Autodesk Inventor part; units mm, degrees
ref_plane "YZ Plane" through (0, 0, 0) normal (1, 0, 0) x (0, 1, 0)
ref_plane "XZ Plane" through (0, 0, 0) normal (0, 1, 0) x (-1, 0, 0)
ref_plane "XY Plane" through (0, 0, 0) normal (0, 0, 1) x (1, 0, 0)
sketch "Sketch1" plane through (0, 0, 0) normal (0, 1, 0) x (-1, 0, 0)
  line L0 (3, 9) -> (-3, 9)
  line L1 (-3, 9) -> (-3, -9)
  line L2 (-3, -9) -> (3, -9)
  line L3 (3, -9) -> (3, 9)
  line L4 (3, 9) -> (-3, -9) construction
  line L5 (-3, 9) -> (3, -9) construction
  circle A0 centre (0, 9) radius 3
  circle A1 centre (0, -9) radius 3
  line L6 (-3, -9) -> (-7, -9)
  line L7 (-7, -9) -> (-7, -5)
  line L8 (-7, -5) -> (-7, -3)
  line L9 (-7, -3) -> (-3, -3)
  line L10 (-7, -3) -> (-7, -6)
  circle A2 centre (-7, -6) radius 3
  line L11 (-3, -3) -> (-3, -9)
  point P0 (0, 0)
  dimension "d0" = 6
  dimension "d1" = 18
  dimension "d2" = 6
  dimension "d4" = 6
  dimension "d5" = 4
  dimension "d6" = 4
  dimension "d7" = 2
  dimension "d10" = 3
  dimension "d11" = 6
extrude "Extrusion1" add sketch "Sketch1" along normal blind 1.5 contours A0 L0 | L0 A0 | L3 A1 L1 A0 | A1 L2 | L2 A1 | A2 L7 L8 | L8 L7 A2
sketch "Sketch2" plane through (0, 1.5, 0) normal (0, 1, 0) x (1, 0, 0)
  line L0 (3, -9) -> (3, 9)
  arc A0 (3, 9) -> (-3, 9) centre (0, 9) ccw
  line L1 (-3, 9) -> (-3, -9)
  arc A1 (-3, -9) -> (3, -9) centre (0, -9) ccw
  circle A2 centre (0, 9) radius 1.5
  circle A3 centre (0, -9) radius 1.5
  line L2 (3, 9) -> (7, 9)
  line L3 (7, 9) -> (7, 3)
  line L4 (7, 3) -> (3, 3)
  line L5 (3, 3) -> (3, 9)
  point P0 (0, 0)
  dimension "d14" = 3
  dimension "d15" = 3
  dimension "d16" = 4
  dimension "d17" = 6
extrude "Extrusion2" cut sketch "Sketch2" against normal blind 1.5 contours L0 L2 L3 L4 | A2 | A3
sketch "Sketch3" plane through (0, 1.5, 0) normal (0, 1, 0) x (1, 0, 0)
  line L0 (3, -9) -> (3, 9)
  arc A0 (3, 9) -> (-3, 9) centre (0, 9) ccw
  line L1 (-3, 9) -> (-3, -9)
  line L2 (3, 9) -> (7, 9)
  line L3 (7, 9) -> (7, 3)
  line L4 (7, 3) -> (3, 3)
  line L5 (3, 3) -> (3, 9)
  point P0 (0, 0)
  dimension "d20" = 4
  dimension "d21" = 6
  dimension "d22" = 4
extrude "Extrusion3" add sketch "Sketch3" against normal blind 1.5
sketch "Sketch4" plane through (0, 1.5, 0) normal (0, 1, 0) x (1, 0, 0)
  arc A0 (7, 3) -> (7, 9) centre (7, 6) ccw
  circle A1 centre (7, 6) radius 1.5
  point P0 (0, 0)
  dimension "d25" = 3
extrude "Extrusion4" cut sketch "Sketch4" against normal blind 1.5
sketch "Sketch5" plane through (0, 0, 0) normal (0, -1, 0) x (1, 0, 0)
  circle A0 centre (7, -6) radius 1.5
  circle A1 centre (0, 9) radius 1.5
  circle A2 centre (0, -9) radius 1.5
  arc A3 (7, -9) -> (7, -3) centre (7, -6) ccw
  arc A4 (3, 9) -> (-3, 9) centre (0, 9) ccw
  arc A5 (-3, -9) -> (3, -9) centre (0, -9) ccw
  circle A6 centre (0, 9) radius 0.1
  circle A7 centre (0, -9) radius 0.1
  circle A8 centre (7, -6) radius 0.1
  point P0 (0, 0)
  dimension "d28" = 0.2
  dimension "d29" = 0.2
  dimension "d30" = 0.2
extrude "Extrusion5" add sketch "Sketch5" against normal blind 1.5
properties part number "tahlo3_sablona"
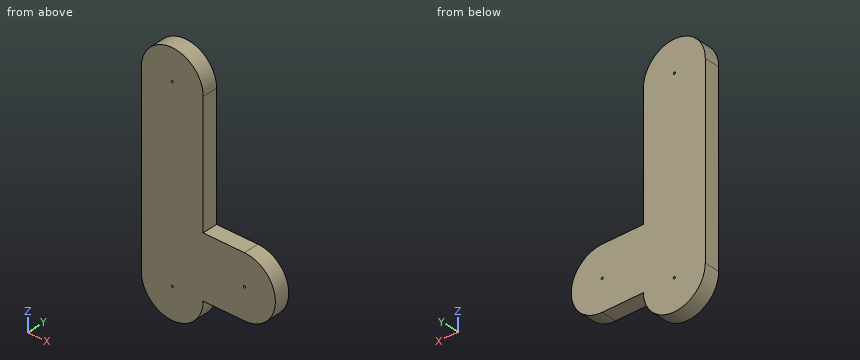
Read the model definition and answer for the solid it produces. Units are mm, in the model's axes. Coordinates: 2 decimals unless noted, no trailing zeros. Loops run counter-clockwise (first coordinate to the right, second up) from the corner with the lowest first, then second, coordinate; pieces in that order, holes last. Notation, with made-up numbers: (68.5, -0.75) - (87.5, -0.75) arc R27 cw to (87.5, 21.25) - close; hole circle Ø3 at (-3, -5). An arc over 180 degrees is marked (long way). Answer in a Markdown table with one row per item.
Q1. Find section C-C on x = 6.25. Write down the section's boundary in (y, z).
Here are the results:
| item | result |
|---|---|
| outline | (0, -9) - (1.5, -9) - (1.5, -3) - (0, -3) - close |
Q2. Given P1, Ø0.8, axis at x = 6, y = 0.5, coming from the -Z side; P2, Ø3, axis at x = 2.5, z = 6, coming from the -Y side, each flat-ended and moving along its own axis, determine where each tip first touches the part or whether it passes through.
Here are the results:
| item | result |
|---|---|
| P1 | stops at z = -9 |
| P2 | stops at y = 0 |
Q3. Straight lines are drawn through the part: line 1 along Z through (x, y) = (0, 0.5); line 2 along Z through (x, y) = (7, 0.6); line 3 along X through (y, z) = (0.95, 9). For each, find the intervals that lie inside material, in ascending order. Write a range as [from, to].
Here are the results:
| item | result |
|---|---|
| line 1 | z = [-12, -9.1], [-8.9, 8.9], [9.1, 12] |
| line 2 | z = [-9, -6.1], [-5.9, -3] |
| line 3 | x = [-3, -0.1], [0.1, 3] |
Q4. Find section A-A on y = 0.75. Write down the section's boundary in (x, z), plus the area to 3 significant figures.
Here are the results:
| item | result |
|---|---|
| outline | (-3, -9) arc R3 ccw to (3, -9) - (7, -9) arc R3 ccw to (7, -3) - (3, -3) - (3, 9) arc R3 ccw to (-3, 9) - close; hole circle Ø0.2 at (0, -9); hole circle Ø0.2 at (0, 9); hole circle Ø0.2 at (7, -6) |
| area | 174 mm^2 |
Q5. Find section B-B on z = 5. Write down the section's boundary in (x, y).
Here are the results:
| item | result |
|---|---|
| outline | (-3, 0) - (3, 0) - (3, 1.5) - (-3, 1.5) - close |
